CAD build for the part. Positions are in the model's coordinates, mm. A direction names the side the tool comes from. Coordinates: 2 decimals unless noted, no trailing zeros. Loops run counter-clockwise (first coordinate to the right, second up) from the corner with the lowest first, then second, coordinate; pieces in that order, holes last. Notation, with made-up numbers: M 10.5,76 L 63.5,76 A23 cw 63.5,91 Z; hole C 70.25,46 d7. An arc over 180 degrees is marked long. Answer as a JSON object with one key per item and string values. Group by question number.
```python
from build123d import *

# Parameters (mm, degrees)
SKETCH_W             = 47.4
SKETCH_H             = 13
SKETCH_R             = 1.65
PAD_DEPTH            = 10
SKETCH001_R          = 3.75
POCKET_DEPTH         = 3.5
SKETCH002_W          = 15.5
SKETCH002_H          = 10
POCKET001_DEPTH      = 100
POCKET001_DEPTH_BACK = -4
SKETCH003_R          = 1.65
POCKET002_DEPTH      = 5.501
POCKET002_DEPTH_BACK = -7.501
POCKET003_DEPTH      = 5.501
POCKET003_DEPTH_BACK = -7.501
POCKET004_DEPTH      = 2.201
SKETCH006_W          = 10
SKETCH006_H          = 10
POCKET005_DEPTH      = 100
POCKET005_DEPTH_BACK = -2.75


with BuildPart() as part:
    # Sketch → Pad (new body)
    with BuildSketch(Plane.XY):
        with Locations((0, -1)):
            Rectangle(SKETCH_W, SKETCH_H)
        with Locations((-20.5, 0)):
            Circle(SKETCH_R, mode=Mode.SUBTRACT)
        with Locations((20.5, 0)):
            Circle(SKETCH_R, mode=Mode.SUBTRACT)
    extrude(amount=-PAD_DEPTH)

    # Sketch001 → Pocket (cut)
    with BuildSketch(Plane.XY):
        with Locations((-20.481411, -0.058129)):
            Circle(SKETCH001_R)
        with Locations((20.5, 0)):
            Circle(SKETCH001_R)
    extrude(amount=-POCKET_DEPTH, mode=Mode.SUBTRACT)

    # Sketch002 → Pocket001 (cut, two sides)
    with BuildSketch(Plane.XZ) as pocket001_sk:
        with Locations((5.6, -5)):
            Rectangle(SKETCH002_W, SKETCH002_H)
    extrude(amount=-POCKET001_DEPTH, mode=Mode.SUBTRACT)
    extrude(pocket001_sk.sketch, amount=-POCKET001_DEPTH_BACK, mode=Mode.SUBTRACT)

    # Sketch003 → Pocket002 (cut, two sides)
    with BuildSketch(Plane.XZ) as pocket002_sk:
        with Locations((-15.5, -5)):
            Circle(SKETCH003_R)
        with Locations((15.5, -5)):
            Circle(SKETCH003_R)
    extrude(amount=-POCKET002_DEPTH, mode=Mode.SUBTRACT)
    extrude(pocket002_sk.sketch, amount=-POCKET002_DEPTH_BACK, mode=Mode.SUBTRACT)

    # Sketch004 → Pocket003 (cut, two sides)
    with BuildSketch(Plane.XZ) as pocket003_sk:
        Polygon((-20.2, 0), (-23.7, -3.5), (-23.7, 0), align=None)
        Polygon((20.2, 0), (23.7, 0), (23.7, -3.5), align=None)
    extrude(amount=-POCKET003_DEPTH, mode=Mode.SUBTRACT)
    extrude(pocket003_sk.sketch, amount=-POCKET003_DEPTH_BACK, mode=Mode.SUBTRACT)

    # Sketch005 (on DatumPlane) → Pocket004 (cut, through all)
    with BuildSketch(Plane.XZ.offset(5.3)):
        Polygon((-13.840118, -7.875), (-12.180236, -5), (-13.840118, -2.125), (-17.159882, -2.125), (-18.819764, -5), (-17.159882, -7.875), align=None)
        Polygon((17.159882, -7.875), (18.819764, -5), (17.159882, -2.125), (13.840118, -2.125), (12.180236, -5), (13.840118, -7.875), align=None)
    extrude(amount=POCKET004_DEPTH, mode=Mode.SUBTRACT)

    # Sketch006 → Pocket005 (cut, two sides)
    with BuildSketch(Plane.XZ) as pocket005_sk:
        with Locations((-8.35, -5)):
            Rectangle(SKETCH006_W, SKETCH006_H)
    extrude(amount=-POCKET005_DEPTH, mode=Mode.SUBTRACT)
    extrude(pocket005_sk.sketch, amount=-POCKET005_DEPTH_BACK, mode=Mode.SUBTRACT)


solid = part.part
```
Item 1: Slice it at B-B, the plane z = -5.75. Count the separate pieces of the cut face and the enclosed holes in it, then the cut area to 3 significant figures.
Item 2: Slice it at D-D, the plane y = 0. Write the cut outline in (x, z), then the cut area to 3 significant figures.
Item 3: Slice it at A-A, the plane y = 4.25. Write the cut outline in (x, z), then the cut area to 3 significant figures.
Item 4: Slice it at C-C, the plane x = -15. Write the cut outline in (y, z) (3 decimals).
Item 5: Tool access for faces 4 (the flat face through (5, -4, -5)), 5 (the cylindrical face through (16.752, 0.136, -1.725)), 6 (the flat face through (-16, -6, -7.875)): list every direction of +Z, -Z, +X, -X, +Y, -Y with a clear straight run to the whole face (end or side of a thin tool).
Item 6: Drill centre lines: L1, parallel to X at y = 0, z = -2.25; L2, parallel to X at y = -2, z = -8.5; L3, parallel to Y at x = 20.5, z = -6.25. Where is each one in solid material? Low to high. Write a range as from..to.
Item 7: Pin check, flat tips, straight feed: pin 1 (4.5 mm diameter, centred on x = 16, z = -5, fed in from -Y); pin 2 (7 mm diameter, centred on x = -20.48, y = -0.06, fed in from +Z). Stop position of each tip, or through.
Item 8: Pull direction Y, two halves, no side cores. Call faces 1 (the flat face through (-18.7, 0, -3.5)), 2 (the flat face through (-8, -2.75, -5)), 3 (the flat face through (13.35, 1, -5)): released by +Y, released by -Y, zero draft, split by the parting line, or undercut.
Computed:
{
 "1": {"separate pieces": "3", "enclosed holes": "2", "area": "280 mm2"},
 "2": {"outline": "M -23.7,-10 L -22.15,-10 L -22.15,-3.5 L -23.7,-3.5 Z; M -18.85,-10 L -13.35,-10 L -13.35,0 L -16.73,0 L -16.73,-3.5 L -18.85,-3.5 Z; M -3.35,-10 L -2.15,-10 L -2.15,0 L -3.35,0 Z; M 13.35,-10 L 18.85,-10 L 18.85,-3.5 L 16.75,-3.5 L 16.75,0 L 13.35,0 Z; M 22.15,-10 L 23.7,-10 L 23.7,-3.5 L 22.15,-3.5 Z; hole C -15.5,-5 d3.3; hole C 15.5,-5 d3.3", "area": "110 mm2"},
 "3": {"outline": "M -23.7,-10 L -13.35,-10 L -13.35,0 L -20.2,0 L -23.7,-3.5 Z; M -3.35,-10 L -2.15,-10 L -2.15,0 L -3.35,0 Z; M 13.35,-10 L 23.7,-10 L 23.7,-3.5 L 20.2,0 L 13.35,0 Z; hole C -15.5,-5 d3.3; hole C 15.5,-5 d3.3", "area": "190 mm2"},
 "4": {"outline": "M -7.5,-10 L 5.5,-10 L 5.5,-6.572 L -5.3,-6.572 L -5.3,-7.875 L -7.5,-7.875 Z; M -7.5,-2.125 L -5.3,-2.125 L -5.3,-3.428 L 5.5,-3.428 L 5.5,0 L -7.5,0 Z"},
 "5": {"face 4": "+Z, -Z, +Y", "face 5": "+Z", "face 6": "-Y"},
 "6": {"L1": "-16.73..-13.35, -3.35..-2.15, 13.35..16.75", "L2": "-23.7..-13.35, -3.35..-2.15, 13.35..23.7", "L3": "-7.5..-1.65, 1.65..5.5"},
 "7": {"pin 1": "y = -5.3", "pin 2": "z = -3.5"},
 "8": {"face 1": "undercut", "face 2": "released by +Y", "face 3": "zero draft"}
}
